Build history of the part. All positions in model axes, mm. Round coordinates to 2 decimals unless told otherwise and drop trailing zeros. Write each loop counter-clockwise with the first axis right and the second up, starting at its lowest first coordinate (ties: lowest second). Pieces come first, ordered by that corner, then holes.
1) Saw through at A-A (y = -40). Write the cut outline in (x, z), plus the area to 3 significant figures.
2) Saw through at D-D (y = 40). Write the cut outline in (x, z).
3) Wall check: probe 1 along X at (y, z) = (-32.5, 8.25); probe 2 along X at (y, z) = (-43, 7); probe 3 along X at (y, z) = (52, 1). Give the ranges that are in metal, low to high.
4) Saw through at C-C (x = -105). Write the cut outline in (y, z).
5) Saw through at B-B (z = 3.25). Write the cut outline in (x, y).
6) Flat gauge pins, fed straight in: pin 1 (10 mm diameter, centred on x = -136.5, y = 37, fed in from +Z); pin 2 (6 mm diameter, centred on y = 31, z = 7, fed in from +X); pin 3 (5 mm diameter, centred on y = 15, z = 4.5, fed in from +X). Where does each tip first touch, or does it go through?
from build123d import *

# Parameters (mm, degrees)
SKETCH1_W           = 1050
SKETCH1_H           = 160
BOSS_EXTRUDE1_DEPTH = 10
SKETCH2_R           = 10
SKETCH2_R_2         = 15
CUT_EXTRUDE3_DEPTH  = 5
FILLET1_R           = 90
FILLET2_R           = 90
SKETCH3_W           = 260
SKETCH3_H           = 160
CUT_EXTRUDE4_DEPTH  = 0.5
SKETCH4_W           = 40
SKETCH4_H           = 160
BOSS_EXTRUDE2_DEPTH = 0.25
SKETCH5_W           = 260
SKETCH5_H           = 9.5
CUT_EXTRUDE5_DEPTH  = 30
SKETCH6_W           = 40
SKETCH6_H           = 30
CUT_EXTRUDE7_DEPTH  = 30
FILLET3_R           = 20
FILLET4_R           = 20


with BuildPart() as part:
    # Sketch1 → Boss-Extrude1 (new body)
    with BuildSketch(Plane.XY):
        Rectangle(SKETCH1_W, SKETCH1_H)
    extrude(amount=BOSS_EXTRUDE1_DEPTH)

    # Sketch2 → Cut-Extrude3 (cut)
    with BuildSketch(Plane.XY.offset(10)):
        with Locations((-135, 40)):
            Circle(SKETCH2_R)
        with Locations((135, 40)):
            Circle(SKETCH2_R)
        with Locations((135, -40)):
            Circle(SKETCH2_R_2)
        with Locations((-135, -40)):
            Circle(SKETCH2_R_2)
    extrude(amount=-CUT_EXTRUDE3_DEPTH, mode=Mode.SUBTRACT)

    # Fillet1
    fillet1_edges = [part.edges().sort_by_distance(p)[0] for p in [
        (525, 80, 5),
    ]]
    fillet(fillet1_edges, radius=FILLET1_R)

    # Fillet2
    fillet2_edges = [part.edges().sort_by_distance(p)[0] for p in [
        (-525, 80, 5),
    ]]
    fillet(fillet2_edges, radius=FILLET2_R)

    # Sketch3 → Cut-Extrude4 (cut)
    with BuildSketch(Plane(origin=(0, 0, 0), x_dir=(-1, 0, 0), z_dir=(0, 0, -1))):
        Rectangle(SKETCH3_W, SKETCH3_H)
    extrude(amount=-CUT_EXTRUDE4_DEPTH, mode=Mode.SUBTRACT)

    # Sketch4 → Boss-Extrude2 (add)
    with BuildSketch(Plane(origin=(0, 0, 0.5), x_dir=(-1, 0, 0), z_dir=(0, 0, -1))):
        Rectangle(SKETCH4_W, SKETCH4_H)
    extrude(amount=BOSS_EXTRUDE2_DEPTH)

    # Sketch5 → Cut-Extrude5 (cut)
    with BuildSketch(Plane(origin=(0, 80, 0), x_dir=(1, 0, 0), z_dir=(0, 1, 0))):
        with Locations((0, -5.25)):
            Rectangle(SKETCH5_W, SKETCH5_H)
    extrude(amount=-CUT_EXTRUDE5_DEPTH, mode=Mode.SUBTRACT)

    # Sketch6 → Cut-Extrude7 (cut)
    with BuildSketch(Plane(origin=(0, 0, 0.25), x_dir=(-1, 0, 0), z_dir=(0, 0, -1))):
        with Locations((0, 65)):
            Rectangle(SKETCH6_W, SKETCH6_H)
    extrude(amount=-CUT_EXTRUDE7_DEPTH, mode=Mode.SUBTRACT)

    # Fillet3
    fillet3_edges = [part.edges().sort_by_distance(p)[0] for p in [
        (130, 80, 5),
    ]]
    fillet(fillet3_edges, radius=FILLET3_R)

    # Fillet4
    fillet4_edges = [part.edges().sort_by_distance(p)[0] for p in [
        (-130, 80, 5),
    ]]
    fillet(fillet4_edges, radius=FILLET4_R)


solid = part.part
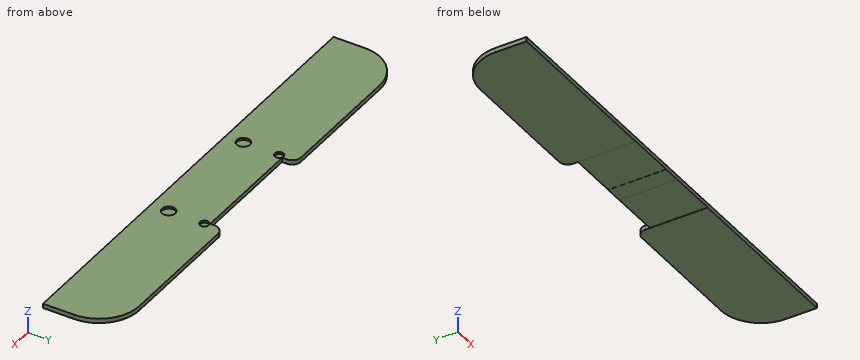
Evaluation:
1. outline: (-525, 0) - (-130, 0) - (-130, 0.5) - (-20, 0.5) - (-20, 0.25) - (20, 0.25) - (20, 0.5) - (130, 0.5) - (130, 0) - (525, 0) - (525, 10) - (150, 10) - (150, 5) - (120, 5) - (120, 10) - (-120, 10) - (-120, 5) - (-150, 5) - (-150, 10) - (-525, 10) - close
1. area: 10,100 mm2
2. outline: (-509.83, 0) - (-130, 0) - (-130, 0.5) - (-20, 0.5) - (-20, 0.25) - (20, 0.25) - (20, 0.5) - (130, 0.5) - (130, 0) - (509.83, 0) - (509.83, 10) - (145, 10) - (145, 5) - (125, 5) - (125, 10) - (-125, 10) - (-125, 5) - (-145, 5) - (-145, 10) - (-509.83, 10) - close
3. probe 1: x = -525 to -147.99, -122.01 to 122.01, 147.99 to 525
3. probe 2: x = -525 to -149.7, -120.3 to 120.3, 149.7 to 525
3. probe 3: x = -500.24 to -130, 130 to 500.24
4. outline: (-80, 0.5) - (50, 0.5) - (50, 10) - (-80, 10) - close
5. outline: (-525, -80) - (525, -80) - (525, -10) arc R90 ccw to (435, 80) - (150, 80) arc R20 ccw to (130, 60) - (130, 50) - (-130, 50) - (-130, 60) arc R20 ccw to (-150, 80) - (-435, 80) arc R90 ccw to (-525, -10) - close
6. pin 1: stops at z = 5
6. pin 2: stops at x = 516.58
6. pin 3: stops at x = 522.14
